from build123d import *

# Parameters (mm, degrees)
SKETCH1_R               = 73.3171
BOSS_EXTRUDE1_DEPTH     = 3.175
F_1_4_CLEARANCE_HOLE1_D = 6.5278
SKETCH4_W               = 100.99999993
SKETCH4_H               = 100.99999993
CUT_EXTRUDE1_DEPTH      = 1
CUT_EXTRUDE1_DEPTH_BACK = 4.175


with BuildPart() as part:
    # Sketch1 → Boss-Extrude1 (new body)
    with BuildSketch(Plane.XY):
        Circle(SKETCH1_R)
    extrude(amount=BOSS_EXTRUDE1_DEPTH)

    # 1/4 Clearance Hole1 (through all)
    with Locations(Plane.XY.offset(3.175)):
        with Locations((-60.325, 0), (60.325, 0)):
            Hole(F_1_4_CLEARANCE_HOLE1_D / 2)

    # Sketch4 → Cut-Extrude1 (cut, two sides)
    with BuildSketch(Plane.XY.offset(3.175)) as cut_extrude1_sk:
        Rectangle(SKETCH4_W, SKETCH4_H)
    extrude(amount=CUT_EXTRUDE1_DEPTH, mode=Mode.SUBTRACT)
    extrude(cut_extrude1_sk.sketch, amount=-CUT_EXTRUDE1_DEPTH_BACK, mode=Mode.SUBTRACT)


solid = part.part
Check sheet for the modelled part. Datum: model origin and axes. Units: mm. A direction names the side the tool comes from. Give positions to 0.01 mm unless a question says otherwise; leave off trailing zeros. Loops run counter-clockwise (first coordinate to the right, second up) from the corner with the lowest first, then second, coordinate; pieces in that order, holes last. Notation, with made-up numbers: M 14.25,53 L 67.25,53 A20 cw 67.25,60 Z; hole C 44.5,24 d2. An arc over 180 degrees is marked long. Use a Markdown table: item, result. Add a question column.
Q1. Sectioned sample at D-D, the plane y = -47. Record the cut outline in (x, z) (3 decimals).
Q2. Go/stop test with flat-tipped pins: pin 1 (6 mm diameter, centred on x = 60.325, y = 0, fed in from -Z); pin 2 (1.5 mm diameter, centred on x = 23, z = 1.5, fed in from +Y); pin 3 (1 mm diameter, centred on x = -28, z = 1, fed in from -Y); pin 4 (1 mm diameter, centred on x = 10, z = 2, fed in from +Y). Record where each tip stops, or that it passes through.
Q3. Sectioned sample at C-C, the plane z = 0.75. Record the cut outline in (x, y) (3 decimals), then the cut area to 3 significant figures.
Q4. Tool access check on faces 4 (the flat face through (5, -54, 0)), 5 (the flat face through (-1, -50.5, 2)). Record the directions out of +Z, -Z, +X, -X, +Y, -Y that give a thin tool (end or side, any length) a straight path to the whole face; none if there is none.
Q5. Sectioned sample at B-B, the plane x = 0. Record the cut outline in (y, z) (3 decimals), then the cut area to 3 significant figures.
Q6. Sectioned sample at A-A, the plane y = 0. Record the cut outline in (x, z) (3 decimals), then the cut area to 3 significant figures.
Q7. Scan lines: line 1 along Y through (x, z) = (36, 0.9); line 2 along X through (y, z) = (-7.5, 1.25); line 3 along Y through (x, z) = (9.5, 2.3). Record each from-to range of solid material in increasing order. Write a range as [from, to].
Q8. Mould release check, pull along X, two halves, no side actions. Record for faces 1 (the flat face through (-50.5, -1, 2)), 2 (the flat face through (5, -54, 3.175)), 3 (the cylindrical face through (33.831, -65.045, 1.565)): pulls with the +X half, pulls with the -X half, needs draft (parallel to the pull), parting line crosses it, or undercut.
Verdict:
| question | item | result |
|---|---|---|
| 1 | outline | M -56.271,0 L -50.5,0 L -50.5,3.175 L -56.271,3.175 Z; M 50.5,0 L 56.271,0 L 56.271,3.175 L 50.5,3.175 Z |
| 2 | pin 1 | through |
| 2 | pin 2 | y = 69.86 |
| 2 | pin 3 | y = -67.96 |
| 2 | pin 4 | y = 72.7 |
| 3 | outline | C 0,0 d146.634; hole C -60.325,0 d6.528; hole M -50.5,-50.5 L 50.5,-50.5 L 50.5,50.5 L -50.5,50.5 Z; hole C 60.325,0 d6.528 |
| 3 | area | 6,620 mm^2 |
| 4 | face 4 | -Z, +X, -X, +Y, -Y |
| 4 | face 5 | +Z, -Z |
| 5 | outline | M -73.317,0 L -50.5,0 L -50.5,3.175 L -73.317,3.175 Z; M 50.5,0 L 73.317,0 L 73.317,3.175 L 50.5,3.175 Z |
| 5 | area | 145 mm^2 |
| 6 | outline | M -73.317,0 L -63.589,0 L -63.589,3.175 L -73.317,3.175 Z; M -57.061,0 L -50.5,0 L -50.5,3.175 L -57.061,3.175 Z; M 50.5,0 L 57.061,0 L 57.061,3.175 L 50.5,3.175 Z; M 63.589,0 L 73.317,0 L 73.317,3.175 L 63.589,3.175 Z |
| 6 | area | 103 mm^2 |
| 7 | line 1 | [-63.87, -50.5], [50.5, 63.87] |
| 7 | line 2 | [-72.93, -50.5], [50.5, 72.93] |
| 7 | line 3 | [-72.7, -50.5], [50.5, 72.7] |
| 8 | face 1 | undercut |
| 8 | face 2 | needs draft |
| 8 | face 3 | parting line crosses it |
